Could you check a few things on this drawing? It's one solid part, dimensions in mm from its lowest x, y, z. A direction names the side the tool comes from. Round coordinates to 2 decimals unless told otherwise and drop trailing zeros. Loops run counter-clockwise (first coordinate to the right, second up) from the corner with the lowest first, then second, coordinate; pieces in that order, holes last. Notation, with made-up numbers: (89, -10.75) -> (127, -10.75) arc R21 cw to (127, 10.25) -> close; hole circle Ø5 at (25, 60.5). An arc over 180 degrees is marked (long way). Use CSV: the item, a comma, the result in double quotes. Start each with the question number.
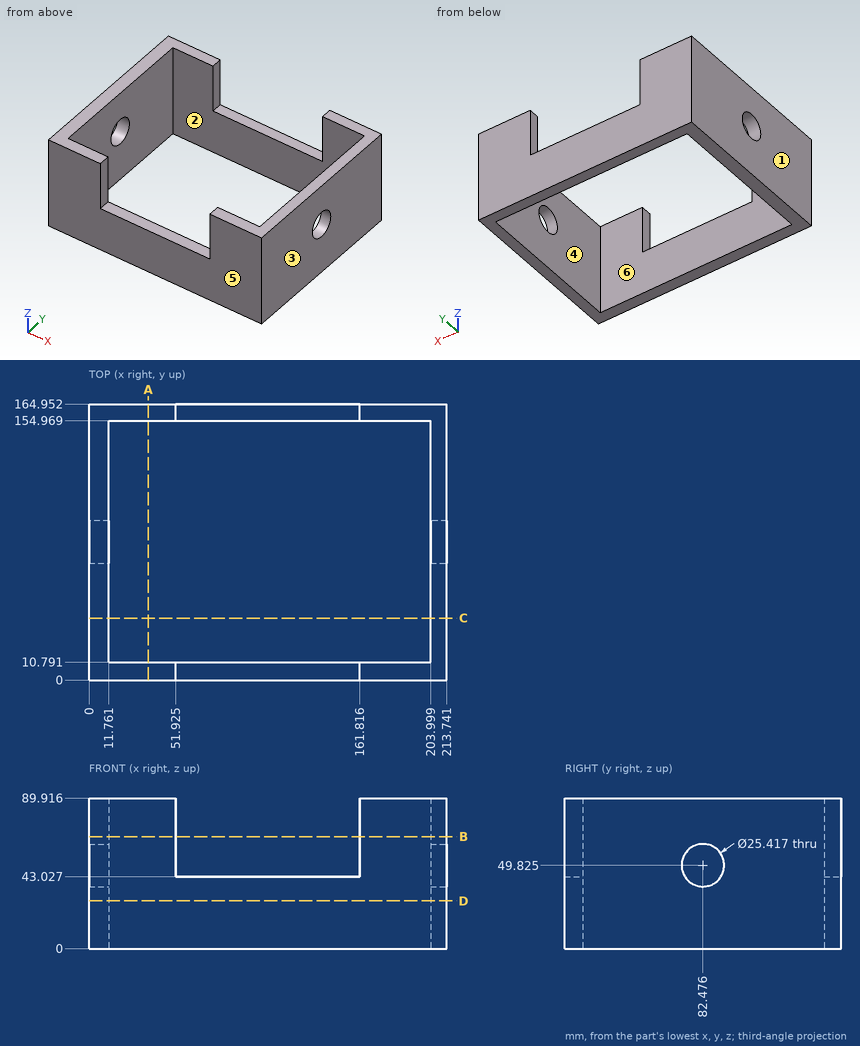
Q1. Will these pins go through, and if not, where does the flat tip stop? pin 1 Ø5.5 at (x, y) = (106.5, 3) entering from +Z; pin 2 Ø15.5 at (y, z) = (82.48, 49.82) entering from -X.
Q2. For the marked faces 5 and 6, which set-ups out of +Z, -Z, +X, -X, +Y, -Y let a thin tool reach every point of the face, with its end or its side?
Q3. I want a section at B-B, the plane z = 67. List the corners of the cut face in (x, y) for me (1 decimal), then the cut area to 3 significant figures.
Q4. I want a section at D-D, the plane z = 28.5. List the corners of the cut face in (x, y) for me, then the cut area to 3 significant figures.
Q5. I need wall thicknesses on line 1 along X through (y, z) = (9, 56) (1 decimal); line 2 along Y through (x, z) = (165, 57); line 3 along X through (y, z) = (68, 67). Which ranges of each line are inside material? Lowest first, please.
Q6. I want a section at C-C, the plane y = 37. List the corners of the cut face in (x, z) for me, then the cut area to 3 significant figures.
Q7. I want a section at A-A, the plane x = 35.5. List the corners of the cut face in (y, z) for me.
Q8. If we mould it in two halves opening along X, with no side actions, what happens to the marked faces 1, 2, 3 and 4? For each: pulls with the +X half, pulls with the -X half, needs draft (parallel to the pull), parting line crosses it, or undercut.
Values found:
1,pin 1,"z = 43.03"
1,pin 2,"through"
2,face 5,"+Z, -Z, +X, -X, -Y"
2,face 6,"+Z, -Z"
3,outline,"(0, 0) -> (51.9, 0) -> (51.9, 10.8) -> (11.8, 10.8) -> (11.8, 155) -> (51.9, 155) -> (51.9, 165) -> (0, 165) -> close; (161.8, 0) -> (213.7, 0) -> (213.7, 165) -> (161.8, 165) -> (161.8, 155) -> (204, 155) -> (204, 10.8) -> (161.8, 10.8) -> close"
3,area,"5,260 mm2"
4,outline,"(0, 0) -> (213.74, 0) -> (213.74, 164.95) -> (0, 164.95) -> close; hole (11.76, 10.79) -> (204, 10.79) -> (204, 154.97) -> (11.76, 154.97) -> close"
4,area,"7,540 mm2"
5,line 1,"0 to 51.9, 161.8 to 213.7"
5,line 2,"0 to 10.79, 154.97 to 164.95"
5,line 3,"0 to 11.76, 204 to 213.74"
6,outline,"(0, 0) -> (11.76, 0) -> (11.76, 89.92) -> (0, 89.92) -> close; (204, 0) -> (213.74, 0) -> (213.74, 89.92) -> (204, 89.92) -> close"
6,area,"1,930 mm2"
7,outline,"(0, 0) -> (10.79, 0) -> (10.79, 89.92) -> (0, 89.92) -> close; (154.97, 0) -> (164.95, 0) -> (164.95, 89.92) -> (154.97, 89.92) -> close"
8,face 1,"pulls with the -X half"
8,face 2,"undercut"
8,face 3,"pulls with the +X half"
8,face 4,"undercut"
